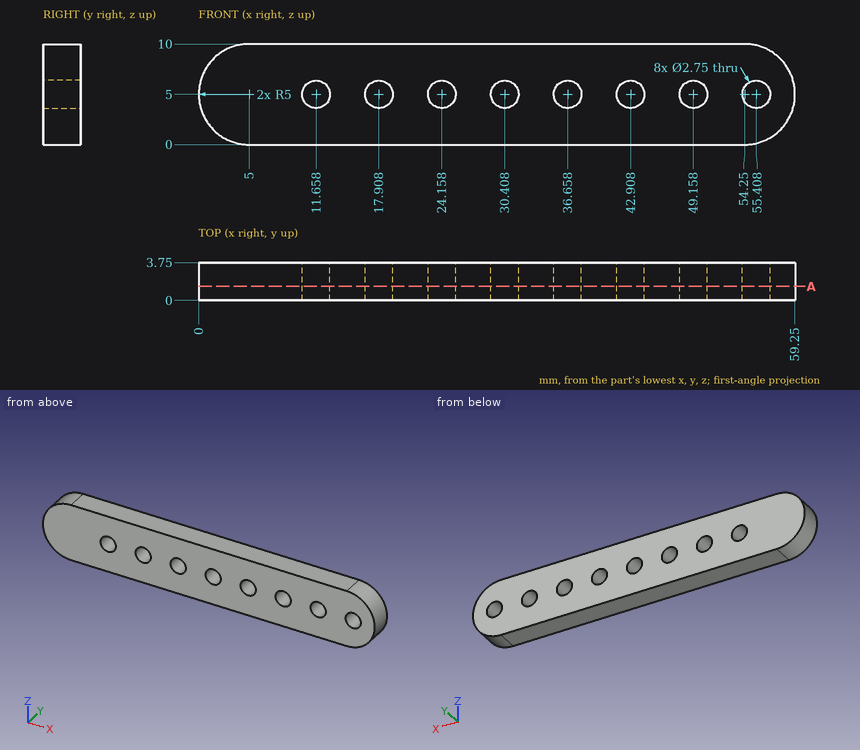
Design review of the part shown in the three views and the two pictorial views. Dimensions are in mm from the part's minimum x, y and z. Round coordinates to 2 decimals unless told otherwise and drop trailing zeros. Answer as a JSON object with one key per item and string values.
1. To check wall thickness, follow line 1 along Z through (x, y) = (36.5, 0.4); line 2 along Z through (x, y) = (48.5, 2.45); line 3 along X through (y, z) = (0.65, 8.25). State the ranges of each line that lie inside material, in increasing order.
Results found:
{"line 1": "z = 0 to 3.63, 6.37 to 10", "line 2": "z = 0 to 3.79, 6.21 to 10", "line 3": "x = 1.2 to 58.05"}
2. Clearance check with a flat-ended pin moving along its axis: pin 1 (1 mm diameter, centred on y = 1.5, z = 1.5, fed in from -X). State where the tip first meets the part, or that it passes through.
Results found:
{"pin 1": "stops at x = 1"}
3. We need section A-A on y = 1.4. State how many separate pieces and enclosed holes the cut face has.
Results found:
{"separate pieces": "1", "enclosed holes": "8"}
